Work out the finished part from the listing and answer in its coordinate system (mm). Round coordinates to 2 decimals unless told otherwise and drop trailing zeros. Order: outer loops, then holes, each group sorted by start corner. A loop starts at its lowest first (then second) coordinate and runs counter-clockwise, first axis right, second up. Notation, with made-up numbers: M -27.5,-21.75 L -4.5,-21.75 A21 ccw -4.5,-13.75 Z; hole C 67,85.25 d3. An arc over 180 degrees is marked long. Return JSON: item names as keys, results as strings.
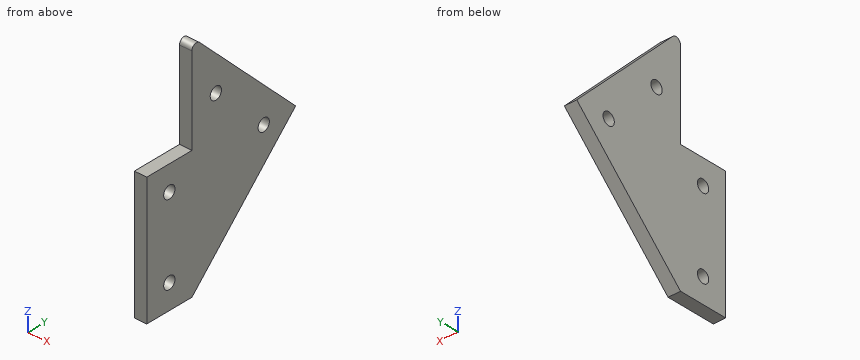
from build123d import *

# Parameters (mm, degrees)
SKETCH_1_R      = 2.5
EXTRUDE_1_DEPTH = 5
FILLET_1_R      = 2


with BuildPart() as part:
    # 草图1 → 凸台-拉伸1 (new body)
    with BuildSketch(Plane(origin=(0, 0, 0), x_dir=(0, 0, -1), z_dir=(1, 0, 0))):
        Polygon((-159.038059223, 45.961940777), (-113.076118446, 0), (-113.076118446, -20), (-165, -20), (-165, 0), (-205, 0), align=None)
        with Locations((-155, -10)):
            Circle(SKETCH_1_R, mode=Mode.SUBTRACT)
        with Locations((-123, -10)):
            Circle(SKETCH_1_R, mode=Mode.SUBTRACT)
        with Locations((-180.251262658, 10.606601718)):
            Circle(SKETCH_1_R, mode=Mode.SUBTRACT)
        with Locations((-159.038059223, 31.819805153)):
            Circle(SKETCH_1_R, mode=Mode.SUBTRACT)
    extrude(amount=EXTRUDE_1_DEPTH)

    # 圆角1
    fillet_1_edges = [part.edges().sort_by_distance(p)[0] for p in [
        (2.5, 0, 205),
    ]]
    fillet(fillet_1_edges, radius=FILLET_1_R)


solid = part.part
Item 1: Find section B-B (z = 154). Determine the outline of the cut face in (x, y).
Output:
{"outline": "M 0,-20 L 5,-20 L 5,-12.29 L 0,-12.29 Z; M 0,-7.71 L 5,-7.71 L 5,40.92 L 0,40.92 Z"}
Item 2: Find section D-D (z = 122.5). Determine the outline of the cut face in (x, y), plus the area to 3 significant figures.
Output:
{"outline": "M 0,-20 L 5,-20 L 5,-12.45 L 0,-12.45 Z; M 0,-7.55 L 5,-7.55 L 5,9.42 L 0,9.42 Z", "area": "123 mm^2"}
Item 3: Each of these flat-tipped pins is pushed along its axis until it touches: pin 1 (1.5 mm diameter, centred on x = 1.5, z = 185.5, fed in from -Y); pin 2 (1 mm diameter, centred on x = 4.5, y = 25.5, fed in from -Z). Where does it stop, or does it pass through?
Output:
{"pin 1": "stops at y = 0", "pin 2": "stops at z = 138.08"}
Item 4: Find section A-A (y = -10). Determine the outline of the cut face in (x, z), plus the area to 3 significant figures.
Output:
{"outline": "M 0,113.08 L 5,113.08 L 5,120.5 L 0,120.5 Z; M 0,125.5 L 5,125.5 L 5,152.5 L 0,152.5 Z; M 0,157.5 L 5,157.5 L 5,165 L 0,165 Z", "area": "210 mm^2"}
Item 5: Find section C-C (z = 173). Determine the outline of the cut face in (x, y), plus the area to 3 significant figures.
Output:
{"outline": "M 0,0 L 5,0 L 5,32 L 0,32 Z", "area": "160 mm^2"}
Item 6: Consider line 1 along Y through (x, z) = (2.45, 155); line 2 along Y through (x, z) = (3.45, 124.5); line 3 along Z through (x, y) = (3.85, -17). Determine where each line is inside the solid, lowest interval first. Write a range as [from, to].
Output:
{"line 1": "y = [-20, -12.5], [-7.5, 41.92]", "line 2": "y = [-20, -12], [-8, 11.42]", "line 3": "z = [113.08, 165]"}
